The model under review builds one solid part; all positions refer to its coordinate system, in mm. A direction names the side the tool comes from. Give positions to 0.01 mm unless a question says otherwise; leave off trailing zeros. Order: outer loops, then holes, each group sorted by start corner. A loop starts at its lowest first (then second) coordinate and runs counter-clockwise, first axis right, second up. Notation, with made-up numbers: M 59,42 L 73,42 A38 ccw 73,81 Z; hole C -30,37 d3. An arc over 180 degrees is marked long. One line per question, with ' | ' between items. Start each with the question number.
1. We need section A-A on z = 5.75. Write out the cut boundary in (x, y).
2. The part is to be moulded in two halves that separate along X. For faces 1 (the face through (3, -12.9, 12)), 2 (the face through (-21.3, 21.1, 12.3)), 3 (the face through (-25.1, 25, 12)), say which applies: +X half, -X half, draft (parallel to the pull), parting line (faces both ways), or undercut.
3. We need section B-B on y = 10. Write out the cut boundary in (x, z), then the cut area to 3 significant figures.
4. Insertion check: P1, Ø2, axis at x = 5.5, z = 3, coming from the -Y side; P2, Ø7.5, axis at y = 15.5, z = 9.5, coming from the -X side; P3, Ø1, axis at x = 5, z = 3, coming from the +Y side. Each pin has a flat end and moves straight along its axis. Give the tip position at first contact, or say it passes through.
5. For faces 4 (the face through (5, 14.6, 2)), 5 (the face through (-20.28, 18.65, 12.32)), 6 (the face through (5, -10.4, 2)), 7 (the face through (5, 2, 5)), list the 3-axis set-ups (+Z, -Z, +X, -X, +Y, -Y) from which the entire face can be reached by the end or side of a thin tool; tool diameter is ignored.
6. We need section D-D on z = 1.5. Write out the cut boundary in (x, y), then the cut area to 3 significant figures.
7. Wall thickness on L1, parallel to X at y = 24, z = 6; L2, parallel to Y at x = -2, z = 9; L3, parallel to X at y = 15.5, z = 19.75: over which ranges is each line inside the solid? List them lowest first.
8. We need section C-C on x = -18. Write out the cut boundary in (y, z).
```python
from build123d import *

# Parameters (mm, degrees)
F1_DEPTH = 25
F0_W     = 2
F0_H     = 25
F2_DEPTH = 5


with BuildPart() as f1:
    # F0 (on Top) → F1 (new body)
    with BuildSketch(Plane.XY):
        Polygon((-19.564466, 19.364466), (-23.1, 22.9), (-23.1, 25.1), (2.1, 25.1), (2.1, -12.9), (4.1, -12.9), (4.1, -10.4), (4.1, 14.6), (4.1, 27.1), (-25.1, 27.1), (-25.1, 22.071573), (-20.97868, 17.950253), align=None)
    extrude(amount=F1_DEPTH)

    # F0 (on Top) → F2 (join)
    with BuildSketch(Plane.XY):
        with Locations((5.1, 2.1)):
            Rectangle(F0_W, F0_H)
    extrude(amount=F2_DEPTH)


solid = f1.part
```
Entries:
1) outline: M -25.1,22.07 L -20.98,17.95 L -19.56,19.36 L -23.1,22.9 L -23.1,25.1 L 2.1,25.1 L 2.1,-12.9 L 4.1,-12.9 L 4.1,27.1 L -25.1,27.1 Z
2) face 1: draft | face 2: undercut | face 3: -X half
3) outline: M 2.1,0 L 6.1,0 L 6.1,5 L 4.1,5 L 4.1,25 L 2.1,25 Z | area: 60.0 mm^2
4) P1: stops at y = -10.4 | P2: stops at x = -22.28 | P3: stops at y = 14.6
5) face 4: +Z, -Z, +X, +Y | face 5: +Z, -Z, -Y | face 6: +Z, -Z, +X, -Y | face 7: +Z, +X, +Y, -Y
6) outline: M -25.1,22.07 L -20.98,17.95 L -19.56,19.36 L -23.1,22.9 L -23.1,25.1 L 2.1,25.1 L 2.1,-12.9 L 4.1,-12.9 L 4.1,-10.4 L 6.1,-10.4 L 6.1,14.6 L 4.1,14.6 L 4.1,27.1 L -25.1,27.1 Z | area: 200 mm^2
7) L1: x = -25.1 to -23.1, 2.1 to 4.1 | L2: y = 25.1 to 27.1 | L3: x = 2.1 to 4.1
8) outline: M 25.1,0 L 27.1,0 L 27.1,25 L 25.1,25 Z
